Autodesk Inventor part; units mm, degrees
ref_plane "YZ Plane" through (0, 0, 0) normal (1, 0, 0) x (0, 1, 0)
ref_plane "XZ Plane" through (0, 0, 0) normal (0, 1, 0) x (-1, 0, 0)
ref_plane "XY Plane" through (0, 0, 0) normal (0, 0, 1) x (1, 0, 0)
sketch "Sketch1" plane through (0, 0, 0) normal (0, 0, 1) x (1, 0, 0)
  line L0 (-2.3, 2.45) -> (2.3, 2.45)
  line L1 (2.3, 2.45) -> (2.3, -2.45)
  line L2 (2.3, -2.45) -> (-2.3, -2.45)
  line L3 (-2.3, -2.45) -> (-2.3, 2.45)
  line L4 (0, 3.43) -> (0, -3.43)
  line L5 (-3.22, 0) -> (3.22, 0)
  point P0 (0, 0)
  dimension "d0" = 4.6
  dimension "d1" = 4.9
extrude "Body" add sketch "Sketch1" against normal blind 8.7
sketch "Sketch2" plane through (0, 0, 0) normal (0, 0, 1) x (1, 0, 0)
  circle A0 centre (0, 0) radius 0.3
  dimension "d4" = 0.6
extrude "Extrusion2" add sketch "Sketch2" along normal blind 3.3
properties part number "Jinlong_Z4TH5B1241992_VibrationMotor_NoHub_Mockup"
CAD build for the part. Positions are in the model's coordinates, mm. Coordinates: 2 decimals unless noted, no trailing zeros. Write each loop counter-clockwise with the first axis right and the second up, starting at its lowest first coordinate (ties: lowest second). Pieces come first, ordered by that corner, then holes. Notation, with made-up numbers: (73, -14) - (123, -14) arc R20 cw to (123, 13) - close; hole circle Ø10 at (53, -6). An arc over 180 degrees is marked (long way). Use a Markdown table: item, result. Add a question column.
Item 1: Band-saw the part on A-A, the plane x = 0. Give the cut face in (y, z).
Item 2: Band-saw the part on C-C, the plane z = 1. Give the cut face in (x, y).
Item 3: Band-saw the part on D-D, the plane x = -0.65. Give the cut face in (y, z), and give its area (3 significant figures).
Item 4: Drill centre line: L1, parallel to Z at x = -1.65, y = 0.8. Where is it in solid material? Low to high. Write a range as from..to.
Item 5: Band-saw the part on B-B, the plane y = 0. Give the cut face in (x, z), and give its area (3 significant figures).
Numbers:
| question | item | result |
|---|---|---|
| 1 | outline | (-2.45, -8.7) - (2.45, -8.7) - (2.45, 0) - (0.3, 0) - (0.3, 3.3) - (-0.3, 3.3) - (-0.3, 0) - (-2.45, 0) - close |
| 2 | outline | circle Ø0.6 at (0, 0) |
| 3 | outline | (-2.45, -8.7) - (2.45, -8.7) - (2.45, 0) - (-2.45, 0) - close |
| 3 | area | 42.6 mm2 |
| 4 | L1 | -8.7..0 |
| 5 | outline | (-2.3, -8.7) - (2.3, -8.7) - (2.3, 0) - (0.3, 0) - (0.3, 3.3) - (-0.3, 3.3) - (-0.3, 0) - (-2.3, 0) - close |
| 5 | area | 42.0 mm2 |
